Geometry check sheet. Reference: the model listing, model coordinates, mm. A direction names the side the tool comes from. Round coordinates to 2 decimals unless told otherwise and drop trailing zeros. Order: outer loops, then holes, each group sorted by start corner. A loop starts at its lowest first (then second) coordinate and runs counter-clockwise, first axis right, second up. Notation, with made-up numbers: (9, -22) - (61, -22) arc R28 cw to (61, 16) - close; hole circle Ø4 at (31, -34.75). An arc over 180 degrees is marked (long way). Use a Markdown table: item, result. Add a question column.
(1) Gauge pin test, flat ends, axial feed: P1, Ø12, axis at x = -3.5, z = 14, coming from the +Y side; P2, Ø10, axis at x = -4, z = 15, coming from the +Y side; P3, Ø3, axis at x = -32.5, z = 17, coming from the -Y side. Record the tip position at first contact, or that the pin passes through.
(2) Access from +Z, -Z, +X, -X, +Y, -Y to the whole of each face (thin tool, end or side, straight path). Record for faces 4 (the face through (28.708, 16.575, 12.522)), 5 (the face through (9.392, -16.575, 12.522)), 6 (the face through (47.492, -16.575, 12.522)).
(3) Thickness scan on line 1 along X through (y, z) = (-18.5, 21.25); line 2 along Y through (x, z) = (32, 14); line 3 along X through (y, z) = (-18, 12). Record the ranges inside material, lowest first. Write a range as [from, to].
(4) Mould release check, pull along Y, two halves, no side actions. Record for faces 1 (the face through (-57.15, 0, 13)), 2 (the face through (9.264, 49.638, 12.522)), 3 (the face through (28.405, 16.693, 12.522)): released by +Y, released by -Y, zero draft, split by the parting line, or undercut.
(5) Section check B-B on x = 33.5. Record the boundary of the cut face in (y, z), then the cut area to 3 significant figures.
(6) Section check C-C on z = 21.5. Give the number of separate pieces and of enclosed holes in the cut face, then the cut area to 3 significant figures.
(7) Section check A-A on y = 48. Record the boundary of the cut face in (x, z).
(8) Section check D-D on x = 3. Record the boundary of the cut face in (y, z) (3 decimals), then the cut area to 3 significant figures.
```python
from build123d import *

# Parameters (mm, degrees)
F1_DEPTH = 25.4
F6_DEPTH = 25.4
F7_DEPTH = 25.4
F8_DEPTH = 25.4
F9_DEPTH = 25.4


with BuildPart() as f1:
    # F0 (on Top) → F1 (new body)
    with BuildSketch(Plane.XY):
        Polygon((19.05, -10.998523), (19.05, 10.998523), (0, 21.997045), (-19.05, 10.998523), (-19.05, -10.998523), (0, -21.997045), align=None)
    extrude(amount=F1_DEPTH)

    # F5 (on Top) → F6 (join)
    with BuildSketch(Plane.XY):
        Polygon((-19.244213, 10.961572), (-0.129696, 21.847583), (0, 43.844246), (-18.984821, 54.954898), (-38.099338, 44.068886), (-38.229034, 22.072224), align=None)
    extrude(amount=F6_DEPTH)

    # F4 (on Top) → F7 (join)
    with BuildSketch(Plane.XY):
        Polygon((-19.05, -10.998523), (-19.05, 10.998523), (-38.1, 21.997045), (-57.15, 10.998523), (-57.15, -10.998523), (-38.1, -21.997045), align=None)
    extrude(amount=F7_DEPTH)

    # F3 (on Top) → F8 (join)
    with BuildSketch(Plane.XY):
        Polygon((19.086355, 11.146432), (37.988951, 22.396404), (37.697487, 44.391519), (18.503427, 55.13666), (-0.399169, 43.886688), (-0.107704, 21.891573), align=None)
    extrude(amount=F8_DEPTH)

    # F2 (on Top) → F9 (join)
    with BuildSketch(Plane.XY):
        Polygon((19.05, 10.998523), (19.05, -10.998523), (38.1, -21.997045), (57.15, -10.998523), (57.15, 10.998523), (38.1, 21.997045), align=None)
    extrude(amount=F9_DEPTH)


solid = f1.part
```
Check sheet entries:
| question | item | result |
|---|---|---|
| 1 | P1 | stops at y = 49.4 |
| 1 | P2 | stops at y = 49.11 |
| 1 | P3 | stops at y = -19.63 |
| 2 | face 4 | +Z, -Z |
| 2 | face 5 | +Z, -Z, -Y |
| 2 | face 6 | +Z, -Z, +X, -Y |
| 3 | line 1 | x = [-44.16, -32.04], [-6.06, 6.06], [32.04, 44.16] |
| 3 | line 2 | y = [-18.48, 18.48], [18.83, 47.58] |
| 3 | line 3 | x = [-45.02, -31.18], [-6.92, 6.92], [31.18, 45.02] |
| 4 | face 1 | zero draft |
| 4 | face 2 | released by +Y |
| 4 | face 3 | undercut |
| 5 | outline | (-19.34, 0) - (19.34, 0) - (19.34, 25.4) - (-19.34, 25.4) - close; (19.72, 0) - (46.74, 0) - (46.74, 25.4) - (19.72, 25.4) - close |
| 5 | area | 1,670 mm2 |
| 6 | separate pieces | 1 |
| 6 | enclosed holes | 2 |
| 6 | area | 6,280 mm2 |
| 7 | outline | (-31.2, 0) - (-7.1, 0) - (-7.1, 25.4) - (-31.2, 25.4) - close; (6.51, 0) - (31.25, 0) - (31.25, 25.4) - (6.51, 25.4) - close |
| 8 | outline | (-20.265, 0) - (45.91, 0) - (45.91, 25.4) - (-20.265, 25.4) - close |
| 8 | area | 1,680 mm2 |
